Geometry: final body of the model. Coordinates: model frame, mm. A direction names the side the tool comes from. Coordinates: 2 decimals unless noted, no trailing zeros. Order: outer loops, then holes, each group sorted by start corner. A loop starts at its lowest first (then second) coordinate and runs counter-clockwise, first axis right, second up. Notation, with made-up numbers: M 38,82.25 L 69,82.25 A8 ccw 69,94.25 Z; hole C 72.25,-4.5 d8. An arc over 180 degrees is marked long. Write item = value, one per line.
from build123d import *

# Parameters (mm, degrees)
SKETCH1_R           = 3.75
SKETCH1_R_2         = 4.5
BOSS_EXTRUDE1_DEPTH = 6.5
CHAMFER1_SIZE       = 1.5


with BuildPart() as part:
    # Sketch1 → Boss-Extrude1 (new body)
    with BuildSketch(Plane.XY):
        with BuildLine():
            Line((-11.458079381, -19.05), (53.381074139, -59.408818568))
            ThreePointArc((53.381074139, -59.408818568), (58.197626483, -59.528635467), (60.641156228, -55.376203052))
            Line((60.641156228, -55.376203052), (60.641156228, 14.3))
            ThreePointArc((60.641156228, 14.3), (59.249913439, 17.658757211), (55.891156228, 19.05))
            Line((55.891156228, 19.05), (-13.723477062, 19.05))
            ThreePointArc((-13.723477062, 19.05), (-14.628464695, 18.040083046), (-15.73121772, 18.829304583))
            ThreePointArc((-15.73121772, 18.829304583), (-17.658815789, 17.658815789), (-18.829304583, 15.73121772))
            ThreePointArc((-18.829304583, 15.73121772), (-18.040083046, 14.628464695), (-19.05, 13.723477062))
            Line((-19.05, 13.723477062), (-19.05, 8.996305235))
            ThreePointArc((-19.05, 8.996305235), (-18.034, 7.980305235), (-19.05, 6.964305235))
            Line((-19.05, 6.964305235), (-19.05, -6.964305235))
            ThreePointArc((-19.05, -6.964305235), (-18.034, -7.980305235), (-19.05, -8.996305235))
            Line((-19.05, -8.996305235), (-19.05, -13.723477062))
            ThreePointArc((-19.05, -13.723477062), (-18.040083046, -14.628464695), (-18.829304583, -15.73121772))
            ThreePointArc((-18.829304583, -15.73121772), (-17.658815789, -17.658815789), (-15.73121772, -18.829304583))
            ThreePointArc((-15.73121772, -18.829304583), (-14.628464695, -18.040083046), (-13.723477062, -19.05))
            Line((-13.723477062, -19.05), (-11.458079381, -19.05))
        make_face()
        with Locations(Location((48.789415314, -34.11185183, 0), (0, 0, 180))):
            Circle(SKETCH1_R, mode=Mode.SUBTRACT)
        with Locations(Location((33.840565899, -24.807012569, 0), (0, 0, 180))):
            Circle(SKETCH1_R, mode=Mode.SUBTRACT)
        with Locations(Location((41.591156228, 0, 0), (0, 0, 180))):
            Circle(SKETCH1_R, mode=Mode.SUBTRACT)
        with Locations(Location((0, 0, 0), (0, 0, 180))):
            Circle(SKETCH1_R_2, mode=Mode.SUBTRACT)
    extrude(amount=BOSS_EXTRUDE1_DEPTH)

    # Chamfer1
    chamfer1_edges = [part.edges().sort_by_distance(p)[0] for p in [
        (-14.628464695, -18.040083046, 6.5),
        (4.5, 0, 6.5),
        (45.341156228, 0, 6.5),
        (37.590565899, -24.807012569, 6.5),
        (52.539415314, -34.11185183, 6.5),
        (-12.590778221, -19.05, 6.5),
        (20.961497379, -39.229409284, 6.5),
        (52.539415314, -34.11185183, 0),
        (37.590565899, -24.807012569, 0),
        (58.197626483, -59.528635467, 6.5),
        (45.341156228, 0, 0),
        (4.5, 0, 0),
        (-17.658815789, -17.658815789, 0),
        (-18.040083046, -14.628464695, 0),
        (-19.05, -11.359891149, 0),
        (-18.034, -7.980305235, 0),
        (-19.05, 0, 0),
        (-18.034, 7.980305235, 0),
        (-19.05, 11.359891149, 0),
        (-18.040083046, 14.628464695, 0),
        (60.641156228, -20.538101526, 6.5),
        (-17.658815789, 17.658815789, 0),
        (-14.628464695, 18.040083046, 0),
        (21.083839583, 19.05, 0),
        (59.249913439, 17.658757211, 0),
        (60.641156228, -20.538101526, 0),
        (58.197626483, -59.528635467, 0),
        (20.961497379, -39.229409284, 0),
        (-12.590778221, -19.05, 0),
        (-14.628464695, -18.040083046, 0),
        (59.249913439, 17.658757211, 6.5),
        (21.083839583, 19.05, 6.5),
        (-14.628464695, 18.040083046, 6.5),
        (-17.658815789, 17.658815789, 6.5),
        (-18.040083046, 14.628464695, 6.5),
        (-19.05, 11.359891149, 6.5),
        (-18.034, 7.980305235, 6.5),
        (-19.05, 0, 6.5),
        (-18.034, -7.980305235, 6.5),
        (-19.05, -11.359891149, 6.5),
        (-18.040083046, -14.628464695, 6.5),
        (-17.658815789, -17.658815789, 6.5),
    ]]
    chamfer(chamfer1_edges, length=CHAMFER1_SIZE)


solid = part.part
1) Section D-D, the plane x = 22.5. Return loops of the section in (y, z).
Numbers:
outline = M -40.19,1.5 L -38.42,0 L 17.55,0 L 19.05,1.5 L 19.05,5 L 17.55,6.5 L -38.42,6.5 L -40.19,5 Z
2) Mould query, pull axis X, two halves, no side actions, for faces 1 (the face through (58.14, -59.56, 3.23)), 2 (the face through (58.62, 16.97, 5.93)), 3 (the face through (3.32, -3.04, 3.23)). Classes: pulls with the +X half, pulls with the -X half, needs draft (parallel to the pull), parting line crosses it, or undercut.
Numbers:
face_1 = parting line crosses it
face_2 = pulls with the +X half
face_3 = undercut
3) Section C-C, the plane z = 3.75. Return loops of the section in (x, y).
Numbers:
outline = M -19.05,-13.72 A1.02 cw -18.83,-15.73 A4.75 ccw -15.73,-18.83 A1.02 cw -13.72,-19.05 L -11.46,-19.05 L 53.38,-59.41 A4.75 ccw 60.64,-55.38 L 60.64,14.3 A4.75 ccw 55.89,19.05 L -13.72,19.05 A1.02 cw -15.73,18.83 A4.75 ccw -18.83,15.73 A1.02 cw -19.05,13.72 L -19.05,9 A1.02 cw -19.05,6.96 L -19.05,-6.96 A1.02 cw -19.05,-9 Z; hole C 0,0 d9; hole C 33.84,-24.81 d7.5; hole C 41.59,0 d7.5; hole C 48.79,-34.11 d7.5
4) Section A-A, the plane y = 0. Return loops of the section in (x, z), and give its area (3 significant figures).
Numbers:
outline = M -19.05,1.5 L -17.55,0 L -6,0 L -4.5,1.5 L -4.5,5 L -6,6.5 L -17.55,6.5 L -19.05,5 Z; M 4.5,1.5 L 6,0 L 36.34,0 L 37.84,1.5 L 37.84,5 L 36.34,6.5 L 6,6.5 L 4.5,5 Z; M 45.34,1.5 L 46.84,0 L 59.14,0 L 60.64,1.5 L 60.64,5 L 59.14,6.5 L 46.84,6.5 L 45.34,5 Z
area = 397 mm²
5) Section B-B, the plane x = 0. Return loops of the section in (y, z), and give its area (3 significant figures).
Numbers:
outline = M -26.18,1.5 L -24.42,0 L -6,0 L -4.5,1.5 L -4.5,5 L -6,6.5 L -24.42,6.5 L -26.18,5 Z; M 4.5,1.5 L 6,0 L 17.55,0 L 19.05,1.5 L 19.05,5 L 17.55,6.5 L 6,6.5 L 4.5,5 Z
area = 226 mm²
6) Set-up query: faces 4 (the face through (-13, -19.05, 3)), 5 (the face through (-14.608, 18.043, 3.226)). Return all of +Z, -Z, +X, -X, +Y, -Y with unobstructed straight access to the full face (end or side cutting, diameter ignored); none if empty.
Numbers:
face_4 = +Z, -Z, -X, -Y
face_5 = +Z, -Z, +Y
7) Line query: L1, parallel to X at y = 0.5, z = 1; L2, parallel to Y at x = 1.5, z = 4.5; L3, parallel to Y at x = 46.5, z = 5.5. Output: solid intervals per line, ascending.
Numbers:
L1 = -18.55 to -4.97, 4.97 to 37.37, 45.81 to 60.14
L2 = -27.12 to -4.24, 4.24 to 19.05
L3 = -54.54 to -37.69, -30.53 to 18.55
8) Pin query (flat end, axial travel): pin 1 (1.1 mm diameter, centred on x = -12.5, z = 3, fed in from -Y); pin 2 (2 mm diameter, centred on y = -29.5, z = 4.5, fed in from -X); pin 3 (1 mm diameter, centred on x = 46, y = -12.5, fed in from -Z); pin 4 (11.5 mm diameter, centred on x = 0, y = 0, fed in from -Z). Return the tip coordinate at first contact, or that it passes through.
Numbers:
pin_1 = -19.05
pin_2 = 3.72
pin_3 = 0
pin_4 = 0.25
